Work out the finished part from the listing and answer in its coordinate system (mm). Give positions to 0.01 mm unless a question says otherwise; leave off trailing zeros. Order: outer loops, then holes, each group sorted by start corner. A loop starts at its lowest first (then second) coordinate and runs counter-clockwise, first axis right, second up. Notation, with made-up numbers: (43, -31) - (92, -31) arc R11 ccw to (92, -12) - close; hole circle Ø1 at (4, 77.25). An arc over 180 degrees is marked (long way). Write each question's results on one line, items separated by ' | '.
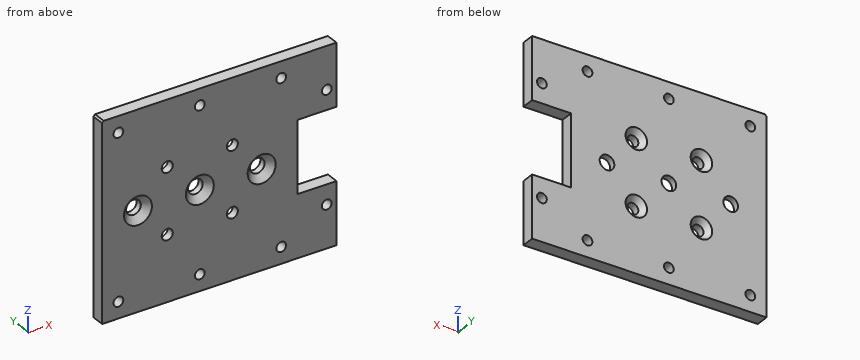
from build123d import *

# Parameters (mm, degrees)
SKETCH_1_W                   = 60
SKETCH_1_H                   = 60
EXTRUDE_1_DEPTH              = 4
HOLE_WIZARD_M3_1_D           = 3.4
HOLE_WIZARD_M3_1_CSINK_D     = 6.6
HOLE_WIZARD_M3_1_CSINK_ANGLE = 90
HOLE_WIZARD_M4_1_AT_2_COUNT  = 2
HOLE_WIZARD_M4_1_AT_2_PITCH  = 19
HOLE_WIZARD_M4_1_AT_3_COUNT  = 2
HOLE_WIZARD_M4_1_AT_3_PITCH  = 38
HOLE_WIZARD_1_D              = 3
SKETCH_9_W                   = 12
SKETCH_9_H                   = 19
SKETCH_9_R                   = 1.5
EXTRUDE_3_DEPTH              = 4
CHAMFER_1_SIZE               = 0.5


with BuildPart() as part:
    # 草图1 → 凸台-拉伸1 (new body)
    with BuildSketch(Plane(origin=(0, 0, 0), x_dir=(1, 0, 0), z_dir=(0, 1, 0))):
        Rectangle(SKETCH_1_W, SKETCH_1_H)
    extrude(amount=EXTRUDE_1_DEPTH)

    # M3 十字槽沉头木螺钉的锥形沉头孔1 (through all)
    with Locations(Plane(origin=(0, 4, 0), x_dir=(1, 0, 0), z_dir=(0, 1, 0))):
        with Locations((-10, 10), (10, 10), (10, -10), (-10, -10)):
            CounterSinkHole(HOLE_WIZARD_M3_1_D / 2, HOLE_WIZARD_M3_1_CSINK_D / 2, counter_sink_angle=HOLE_WIZARD_M3_1_CSINK_ANGLE)

    # 草图5 → M4 十字槽沉头木螺钉的锥形沉头孔1 (revolve, cut)
    with BuildSketch(Plane(origin=(-19, 0, 0), x_dir=(0, 0, -1), z_dir=(1, 0, 0))):
        Polygon((0, 0), (0, 4), (2.25, 4), (2.25, 2.05), (4.3, 0), align=None)
    hole_wizard_m4_1 = revolve(axis=Axis((-19, -6.35, 0), (0, 1, 0)), mode=Mode.SUBTRACT)

    # M4 十字槽沉头木螺钉的锥形沉头孔1 at 2: M4 十字槽沉头木螺钉的锥形沉头孔1 ×2
    with Locations(*[(i * HOLE_WIZARD_M4_1_AT_2_PITCH, 0, 0) for i in range(1, HOLE_WIZARD_M4_1_AT_2_COUNT)]):
        add(hole_wizard_m4_1, mode=Mode.SUBTRACT)

    # M4 十字槽沉头木螺钉的锥形沉头孔1 at 3: M4 十字槽沉头木螺钉的锥形沉头孔1 ×2
    with Locations(*[(i * HOLE_WIZARD_M4_1_AT_3_PITCH, 0, 0) for i in range(1, HOLE_WIZARD_M4_1_AT_3_COUNT)]):
        add(hole_wizard_m4_1, mode=Mode.SUBTRACT)

    # 孔1 (through all)
    with Locations(Plane(origin=(0, 4, 0), x_dir=(1, 0, 0), z_dir=(0, 1, 0))):
        with Locations((25, 25), (25, -25), (0, -25), (-25, -25), (-25, 25), (0, 25)):
            Hole(HOLE_WIZARD_1_D / 2)

    # 草图9 → 凸台-拉伸3 (add)
    with BuildSketch(Plane(origin=(0, 4, 0), x_dir=(1, 0, 0), z_dir=(0, 1, 0))):
        with Locations((36, -20.5)):
            Rectangle(SKETCH_9_W, SKETCH_9_H)
        with Locations(Location((39, -17, 0), (0, 0, 270))):
            Circle(SKETCH_9_R, mode=Mode.SUBTRACT)
    extrude_3 = extrude(amount=-EXTRUDE_3_DEPTH)

    # 倒角1
    chamfer_1_edges = [part.edges().sort_by_distance(p)[0] for p in [
        (-30, 2, 30),
    ]]
    chamfer(chamfer_1_edges, length=CHAMFER_1_SIZE)

    # 镜向1: 凸台-拉伸3 across plane
    add(extrude_3.mirror(Plane.XY))


solid = part.part
1. Straight lines are drawn through the part: line 1 (X direction, y = 2.6, z = 25); line 2 (Z direction, x = 10, y = 1.25); line 3 (Z direction, x = 25, y = 1.25). For each, find the intervals that lie inside material, in ascending order. Write a range as [from, to].
Answer list:
line 1: [-30, -26.5], [-23.5, -1.5], [1.5, 23.5], [26.5, 42] | line 2: [-30, -11.7], [-8.3, 8.3], [11.7, 30] | line 3: [-30, -26.5], [-23.5, 23.5], [26.5, 30]
2. A cutting plane is placed at C-C, the plane z = 25. Write down the section's boundary in (x, y), then the cut area to 3 significant figures.
Answer list:
outline: (-30, 0) - (-26.5, 0) - (-26.5, 4) - (-30, 4) - close; (-23.5, 0) - (-1.5, 0) - (-1.5, 4) - (-23.5, 4) - close; (1.5, 0) - (23.5, 0) - (23.5, 4) - (1.5, 4) - close; (26.5, 0) - (42, 0) - (42, 4) - (26.5, 4) - close | area: 252 mm^2
3. A cutting plane is placed at D-D, the plane y = 3.05. State how many separate pieces and enclosed holes the cut face has, then the cut area to 3 significant figures.
Answer list:
separate pieces: 1 | enclosed holes: 15 | area: 3,880 mm^2
4. Given P1, Ø6, axis at x = -19, z = 0, coming from the -Y side; P2, Ø7, axis at x = 19, z = 0, coming from the -Y side; P3, Ø6, axis at x = 1, z = -0.5, coming from the -Y side, each flat-ended and moving along its own axis, determine where each tip first touches the part or whether it passes through.
Answer list:
P1: y = 1.3 | P2: y = 0.8 | P3: y = 0.18
5. A cutting plane is placed at A-A, the plane x = 25. Write down the section's boundary in (y, z).
Answer list:
outline: (0, -30) - (4, -30) - (4, -26.5) - (0, -26.5) - close; (0, -23.5) - (4, -23.5) - (4, 23.5) - (0, 23.5) - close; (0, 26.5) - (4, 26.5) - (4, 30) - (0, 30) - close
6. A cutting plane is placed at B-B, the plane z = -17. Write down the section's boundary in (x, y), then the cut area to 3 significant figures.
Answer list:
outline: (-30, 0) - (37.5, 0) - (37.5, 4) - (-30, 4) - close; (40.5, 0) - (42, 0) - (42, 4) - (40.5, 4) - close | area: 276 mm^2
